Build history of the part. All positions in model axes, mm. Face numbers are marked on the shaded views. A direction names the side the tool comes from. Round coordinates to 2 decimals unless told otherwise and drop trailing zeros. Loops run counter-clockwise (first coordinate to the right, second up) from the corner with the lowest first, then second, coordinate; pieces in that order, holes last. Notation, with made-up numbers: (17.5, 88) - (21.5, 88) arc R16 ccw to (21.5, 118) - close; hole circle Ø3 at (-21.75, -28.75). An arc over 180 degrees is marked (long way). One line per question, with ' | ' between items. Start each with the question number.
Autodesk Fusion 360 part; units mm, degrees
sketch "Sketch1" plane through (0, 0, 0) normal (0, 0, 1) x (1, 0, 0)
  circle A0 centre (0, 0) radius 48
  dimension "d1" = 96
extrude "Extrude1" add sketch "Sketch1" along normal blind 5
sketch "Sketch2" plane through (0, 0, 5) normal (0, 0, 1) x (-1, 0, 0)
  circle A0 centre (0, 0) radius 48
  circle A1 centre (0, 0) radius 50
extrude "Extrude2" add sketch "Sketch2" along normal blind 2 contours A0 | A1
extrude "Extrude3" add sketch "Sketch1" along normal blind 15
sketch "Sketch3" plane through (0, 0, 15) normal (0, 0, 1) x (-1, 0, 0)
  circle A0 centre (0, 0) radius 48
  line L0 (3.9499, -6.8414) -> (7.8997, 0)
  line L1 (7.8997, 0) -> (3.9499, 6.8414)
  line L2 (3.9499, 6.8414) -> (-3.9499, 6.8414)
  line L3 (-3.9499, 6.8414) -> (-7.8997, 0)
  line L4 (-7.8997, 0) -> (-3.9499, -6.8414)
  line L5 (-3.9499, -6.8414) -> (3.9499, -6.8414)
extrude "Extrude4" add sketch "Sketch3" along normal blind 110 contours L0 L1 L2 L3 L4 L5
sketch "Sketch4" plane through (0, 0, 15) normal (0, 0, 1) x (-1, 0, 0)
  line L0 (-3.9499, -6.8414) -> (-7.8997, 0)
  line L1 (-7.8997, 0) -> (-3.9499, 6.8414)
  line L2 (-3.9499, 6.8414) -> (3.9499, 6.8414)
  line L3 (3.9499, 6.8414) -> (7.8997, 0)
  line L4 (7.8997, 0) -> (3.9499, -6.8414)
  line L5 (3.9499, -6.8414) -> (-3.9499, -6.8414)
  circle A0 centre (0, 0) radius 48
  circle A1 centre (0, 35) radius 5
extrude "Extrude5" cut sketch "Sketch4" against normal blind 15 contours A1
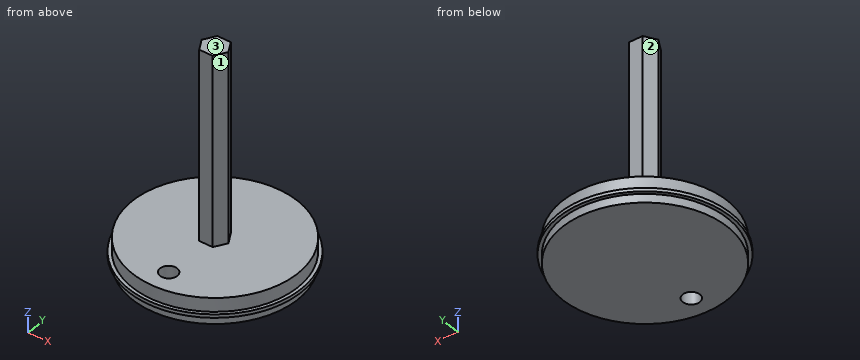
1) Saw through at D-D on y = -35. Write the cut outline in (x, z).
2) Saw through at A-A on x = 0. Write the cut outline in (y, z).
3) Tool access for the marked faces 1, 2 and 3: list every direction of +Z, -Z, +X, -X, +Y, -Y with a clear straight run to the whole face (end or side of a thin tool).
4) Drop flat-ended pins along their axis: pin 1 (10 mm diameter, centred on x = 17.5, z = 53, fed in from -Y); pin 2 (8.5 mm diameter, centred on x = 1.5, z = 67, fed in from +Y); pin 3 (8 mm diameter, centred on x = 34.5, y = -39.5, fed in from -Z); pin 4 (8 mm diameter, centred on x = 2.5, z = 69, fed in from -Y). Give the stop position or say it passes through.
5) Saw through at C-C on y = 13. Write the cut outline in (x, z), and give its area (3 significant figures).
6) Saw through at B-B on z = 49. Write the cut outline in (x, y), and give its area (3 significant figures).
7) Wall check: line 1 (Y direction, x = 0, z = 4.75); line 2 (Z direction, x = -36, y = -29.5); line 3 (Y direction, x = 5, z = 107). Give the ranges that are in metal, low to high. Write a range as [from, to].
Answer key:
1) outline: (-35.71, 5) - (-32.85, 5) - (-32.85, 0) - (-5, 0) - (-5, 15) - (-32.85, 15) - (-32.85, 7) - (-35.71, 7) - close; (5, 0) - (32.85, 0) - (32.85, 5) - (35.71, 5) - (35.71, 7) - (32.85, 7) - (32.85, 15) - (5, 15) - close
2) outline: (-50, 5) - (-48, 5) - (-48, 0) - (-40, 0) - (-40, 15) - (-48, 15) - (-48, 7) - (-50, 7) - close; (-30, 0) - (48, 0) - (48, 5) - (50, 5) - (50, 7) - (48, 7) - (48, 15) - (6.84, 15) - (6.84, 125) - (-6.84, 125) - (-6.84, 15) - (-30, 15) - close
3) face 1: +Z, +X, -Y | face 2: +Z, -X, +Y | face 3: +Z, +X, -X, +Y, -Y
4) pin 1: through | pin 2: y = 6.84 | pin 3: z = 5 | pin 4: y = -6.84
5) outline: (-48.28, 5) - (-46.21, 5) - (-46.21, 0) - (46.21, 0) - (46.21, 5) - (48.28, 5) - (48.28, 7) - (46.21, 7) - (46.21, 15) - (-46.21, 15) - (-46.21, 7) - (-48.28, 7) - close | area: 1,390 mm²
6) outline: (-7.9, 0) - (-3.95, -6.84) - (3.95, -6.84) - (7.9, 0) - (3.95, 6.84) - (-3.95, 6.84) - close | area: 162 mm²
7) line 1: [-48, -40], [-30, 48] | line 2: [0, 15] | line 3: [-5.02, 5.02]
